Source: CAD feature listing. Evaluate the final solid. Frame: model axes, mm. A direction names the side the tool comes from. Coordinates: 2 decimals unless noted, no trailing zeros. Order: outer loops, then holes, each group sorted by start corner. A loop starts at its lowest first (then second) coordinate and runs counter-clockwise, first axis right, second up.
```python
from build123d import *

# Parameters (mm, degrees)
SKETCH1_W           = 609.6
SKETCH1_H           = 165.1
BOSS_EXTRUDE1_DEPTH = 609.6
SHELL1_T            = -6.35
SKETCH2_R           = 44.45
CUT_EXTRUDE2_DEPTH  = 7.62
SKETCH4_W           = 88.9
SKETCH4_H           = 88.9
CUT_EXTRUDE3_DEPTH  = 7.62


with BuildPart() as part:
    # Sketch1 → Boss-Extrude1 (new body)
    with BuildSketch(Plane.XY):
        Rectangle(SKETCH1_W, SKETCH1_H)
    extrude(amount=-BOSS_EXTRUDE1_DEPTH)

    # Shell1
    shell1_openings = [part.faces().sort_by_distance(p)[0] for p in [
        (-304.8, 0, -304.8),
    ]]
    offset(amount=SHELL1_T, openings=shell1_openings, kind=Kind.INTERSECTION)

    # Sketch2 → Cut-Extrude2 (cut)
    with BuildSketch(Plane(origin=(0, 82.55, 0), x_dir=(1, 0, 0), z_dir=(0, 1, 0))):
        with Locations((-212.941456521, 378.528168367)):
            Circle(SKETCH2_R)
        with Locations((-212.941456521, 226.128168367)):
            Circle(SKETCH2_R)
        with Locations((-212.941456521, 73.728168367)):
            Circle(SKETCH2_R)
        with Locations((-9.741456521, 226.128168367)):
            Circle(SKETCH2_R)
        with Locations((-9.741456521, 378.528168367)):
            Circle(SKETCH2_R)
        with Locations((-9.741456521, 73.728168367)):
            Circle(SKETCH2_R)
        with Locations((193.458543479, 226.128168367)):
            Circle(SKETCH2_R)
        with Locations((193.458543479, 378.528168367)):
            Circle(SKETCH2_R)
        with Locations((193.458543479, 73.728168367)):
            Circle(SKETCH2_R)
        with Locations((-212.941456521, 530.928168367)):
            Circle(SKETCH2_R)
        with Locations((-9.741456521, 530.928168367)):
            Circle(SKETCH2_R)
        with Locations((193.458543479, 530.928168367)):
            Circle(SKETCH2_R)
    extrude(amount=-CUT_EXTRUDE2_DEPTH, mode=Mode.SUBTRACT)

    # Sketch4 → Cut-Extrude3 (cut)
    with BuildSketch(Plane(origin=(0, 0, -609.6), x_dir=(-1, 0, 0), z_dir=(0, 0, -1))):
        with Locations((260.35, -31.75)):
            Rectangle(SKETCH4_W, SKETCH4_H)
    extrude(amount=-CUT_EXTRUDE3_DEPTH, mode=Mode.SUBTRACT)


solid = part.part
```
Q1. Section query C-C on z = -563.5. Output: boundary loops of the cut face in (x, y).
Solutions:
outline: (-304.8, -82.55) - (304.8, -82.55) - (304.8, 82.55) - (223.71, 82.55) - (223.71, 76.2) - (298.45, 76.2) - (298.45, -76.2) - (-304.8, -76.2) - close; (-304.8, 76.2) - (-243.19, 76.2) - (-243.19, 82.55) - (-304.8, 82.55) - close; (-182.69, 76.2) - (-39.99, 76.2) - (-39.99, 82.55) - (-182.69, 82.55) - close; (20.51, 76.2) - (163.21, 76.2) - (163.21, 82.55) - (20.51, 82.55) - close
Q2. Section query A-A on y = -6. Output: boundary loops of the cut face in (x, z), plus the area to 3 significant figures.
Solutions:
outline: (-304.8, -6.35) - (298.45, -6.35) - (298.45, -603.25) - (-215.9, -603.25) - (-215.9, -609.6) - (304.8, -609.6) - (304.8, 0) - (-304.8, 0) - close
area: 11,000 mm2
Q3. Section query D-D on x = 194. Output: boundary loops of the cut face in (y, z), plus the area to 3 significant figures.
Solutions:
outline: (-82.55, -609.6) - (82.55, -609.6) - (82.55, -575.37) - (76.2, -575.37) - (76.2, -603.25) - (-76.2, -603.25) - (-76.2, -6.35) - (76.2, -6.35) - (76.2, -29.28) - (82.55, -29.28) - (82.55, 0) - (-82.55, 0) - close; (76.2, -486.48) - (82.55, -486.48) - (82.55, -422.97) - (76.2, -422.97) - close; (76.2, -334.08) - (82.55, -334.08) - (82.55, -270.57) - (76.2, -270.57) - close; (76.2, -181.68) - (82.55, -181.68) - (82.55, -118.17) - (76.2, -118.17) - close
area: 7,420 mm2
Q4. Section query B-B on x = -264.5. Output: boundary loops of the cut face in (y, z), plus the area to 3 significant figures.
Solutions:
outline: (-82.55, -609.6) - (-76.2, -609.6) - (-76.2, -6.35) - (76.2, -6.35) - (76.2, -603.25) - (12.7, -603.25) - (12.7, -609.6) - (82.55, -609.6) - (82.55, 0) - (-82.55, 0) - close
area: 9,110 mm2
Q5. Set-up query: faces 4 (the flat face through (-304.8, 79, -303)), 5 (the cylindrical face through (10.77, 79.419, -339.093)), 6 (the flat face through (-7, 1, -6.35)). Return all of +Z, -Z, +X, -X, +Y, -Y with unobstructed straight access to the full face (end or side cutting, diameter ignored); none if empty.
Solutions:
face 4: +Z, -Z, -X, +Y, -Y
face 5: +Y
face 6: -X
Q6. Pin query (flat end, axial travel): P1, Ø7, axis at y = -40.5, z = -605.5, coming from the -X side; P2, Ø1, axis at y = -3, z = -226, coming from the -X side. Return the tip coordinate at first contact, or that it passes through.
Solutions:
P1: stops at x = -215.9
P2: stops at x = 298.45
Q7. Pull-direction query (Z, two-part tool) for faces 1 (the flat face through (-4, 1, -609.6)), 2 (the cylindrical face through (-45.015, 79.419, -46.681)), 3 (the flat face through (-4, -82.55, -301)); classes: pulls with the +Z half, pulls with the -Z half, needs draft (parallel to the pull), parting line crosses it, or undercut.
Solutions:
face 1: pulls with the -Z half
face 2: undercut
face 3: needs draft
Q8. Material intervals for line 1 along Z through (x, y) = (194.5, -31); line 2 along Y through (x, z) = (-184, -275), sorted ascending.
Solutions:
line 1: z = -609.6 to -603.25, -6.35 to 0
line 2: y = -82.55 to -76.2, 76.2 to 82.55
